from build123d import *

# Parameters (mm, degrees)
SKETCH2_W               = 36
SKETCH2_H               = 36
SKETCH2_R               = 1.5
BOSS_EXTRUDE2_DEPTH     = 1
FILLET1_R               = 0.5
CROQUIS1_R              = 2.1
CROQUIS1_R_2            = 1.5
SALIENTE_EXTRUIR1_DEPTH = 2


with BuildPart() as part:
    # Sketch2 → Boss-Extrude2 (new body)
    with BuildSketch(Plane(origin=(0, 0, 0), x_dir=(1, 0, 0), z_dir=(0, 1, 0))):
        Rectangle(SKETCH2_W, SKETCH2_H)
        with Locations(Location((-15, 15, 0), (0, 0, 270))):
            Circle(SKETCH2_R, mode=Mode.SUBTRACT)
        with Locations(Location((-15, -15, 0), (0, 0, 270))):
            Circle(SKETCH2_R, mode=Mode.SUBTRACT)
        with Locations(Location((15, -15, 0), (0, 0, 270))):
            Circle(SKETCH2_R, mode=Mode.SUBTRACT)
        with Locations(Location((15, 15, 0), (0, 0, 270))):
            Circle(SKETCH2_R, mode=Mode.SUBTRACT)
    extrude(amount=BOSS_EXTRUDE2_DEPTH)

    # Fillet1
    fillet1_edges = [part.edges().sort_by_distance(p)[0] for p in [
        (-18, 1, 0),
        (0, 1, 18),
        (18, 1, 0),
        (0, 0, 18),
        (-18, 0, 0),
        (0, 0, -18),
        (18, 0, 0),
        (0, 1, -18),
        (18, 0.5, 18),
        (-18, 0.5, 18),
        (-18, 0.5, -18),
        (18, 0.5, -18),
    ]]
    fillet(fillet1_edges, radius=FILLET1_R - 0.0001)  # a hair under: the kernel refuses the full size

    # Croquis1 → Saliente-Extruir1 (add)
    # profile 1 of 4: a face of its own
    with BuildSketch(Plane(origin=(0, 1, 0), x_dir=(1, 0, 0), z_dir=(0, 1, 0))):
        with Locations(Location((-15, -15, 0), (0, 0, 90))):
            Circle(CROQUIS1_R)
        with Locations(Location((-15, -15, 0), (0, 0, 270))):
            Circle(CROQUIS1_R_2, mode=Mode.SUBTRACT)
    # profile 2 of 4: a face of its own
    with BuildSketch(Plane(origin=(0, 1, 0), x_dir=(1, 0, 0), z_dir=(0, 1, 0))):
        with Locations(Location((-15, 15, 0), (0, 0, 90))):
            Circle(CROQUIS1_R)
        with Locations(Location((-15, 15, 0), (0, 0, 270))):
            Circle(CROQUIS1_R_2, mode=Mode.SUBTRACT)
    # profile 3 of 4: a face of its own
    with BuildSketch(Plane(origin=(0, 1, 0), x_dir=(1, 0, 0), z_dir=(0, 1, 0))):
        with Locations(Location((15, 15, 0), (0, 0, 90))):
            Circle(CROQUIS1_R)
        with Locations(Location((15, 15, 0), (0, 0, 270))):
            Circle(CROQUIS1_R_2, mode=Mode.SUBTRACT)
    # profile 4 of 4: a face of its own
    with BuildSketch(Plane(origin=(0, 1, 0), x_dir=(1, 0, 0), z_dir=(0, 1, 0))):
        with Locations(Location((15, -15, 0), (0, 0, 90))):
            Circle(CROQUIS1_R)
        with Locations(Location((15, -15, 0), (0, 0, 270))):
            Circle(CROQUIS1_R_2, mode=Mode.SUBTRACT)
    extrude(amount=SALIENTE_EXTRUIR1_DEPTH)


solid = part.part
Part model, mm, in its own coordinate system. A direction names the side the tool comes from. Coordinates: 2 decimals unless noted, no trailing zeros. Loops run counter-clockwise (first coordinate to the right, second up) from the corner with the lowest first, then second, coordinate; pieces in that order, holes last. Notation, with made-up numbers: (42.25, 61.5) -> (74.25, 61.5) arc R16 cw to (74.25, 65.5) -> close; hole circle Ø9 at (-10.5, 41). An arc over 180 degrees is marked (long way). Use a Markdown table: item, result. Add a question column.
Item 1: Pull direction X, two halves, no side cores. Call faces 1 (the flat face through (16.4, 3, -15.9)), 2 (the cylindrical face through (12.918, 1.986, 15.273)): +X half, -X half, draft (parallel to the pull), parting line (faces both ways), or undercut.
Item 2: Flat gauge pins, fed straight in: P1, Ø1, axis at x = 2.5, z = -12.5, coming from the +Y side; P2, Ø3.5, axis at x = -15, z = 15, coming from the -Y side; P3, Ø2.5, axis at x = 15, z = 15, coming from the +Y side. Where does each tip first touch, or does it go through?
Item 3: Band-saw the part on A-A on y = 1.6. Write the cut outline in (x, z), plus the area to 3 significant figures.
Item 4: Band-saw the part on B-B on x = -15. Give the number of separate pieces and of enclosed holes in the cut face, plus the area to 3 significant figures.
Item 5: Which spindle directions (+Z, -Z, +X, -X, +Y, -Y) get a long thin tool onto all of the face, cutting with end or side? Do faces 3 (the cylindrical face through (-14.93, 1.48, 13.5)), 4 (the cylindrical face through (-16.77, 1.99, -16.13)). Say none if no direction does.
Item 6: Probe probe 1 along X at (y, z) = (1.75, -15); probe 2 along X at (y, z) = (0.6, 15); probe 3 along Y at (x, z) = (12.5, -1.5). List the from-to ranges inside material, lowest first.
Geometry says:
| question | item | result |
|---|---|---|
| 1 | face 1 | draft |
| 1 | face 2 | undercut |
| 2 | P1 | y = 1 |
| 2 | P2 | y = 0 |
| 2 | P3 | through |
| 3 | outline | circle Ø4.2 at (-15, -15); circle Ø4.2 at (-15, 15); circle Ø4.2 at (15, -15); circle Ø4.2 at (15, 15); hole circle Ø3 at (-15, -15); hole circle Ø3 at (-15, 15); hole circle Ø3 at (15, -15); hole circle Ø3 at (15, 15) |
| 3 | area | 27.1 mm² |
| 4 | separate pieces | 3 |
| 4 | enclosed holes | 0 |
| 4 | area | 34.6 mm² |
| 5 | face 3 | +Y, -Y |
| 5 | face 4 | +Y |
| 6 | probe 1 | -17.1 to -16.5, -13.5 to -12.9, 12.9 to 13.5, 16.5 to 17.1 |
| 6 | probe 2 | -17.99 to -16.5, -13.5 to 13.5, 16.5 to 17.99 |
| 6 | probe 3 | 0 to 1 |
